Design review of the part built by this model. Coordinates are the model's own, in mm. A direction names the side the tool comes from. Give positions to 0.01 mm unless a question says otherwise; leave off trailing zeros. Order: outer loops, then holes, each group sorted by start corner. A loop starts at its lowest first (then second) coordinate and runs counter-clockwise, first axis right, second up.
```python
from build123d import *

# Parameters (mm, degrees)
SKETCH_1_W          = 38
SKETCH_1_H          = 70
SKETCH_1_R          = 1.5
SKETCH_1_W_2        = 30
SKETCH_1_H_2        = 54
SKETCH_1_H_3        = 5
EXTRUDE_1_DEPTH     = 3
EXTRUDE_2_DEPTH     = 3
FILLET_1_R          = 2
SKETCH_4_R          = 1.5
CUT_EXTRUDE_1_DEPTH = 10
FILLET_2_R          = 5


with BuildPart() as part:
    # 草图1 → 凸台-拉伸1 (new body)
    # profile 1 of 2: a face of its own
    with BuildSketch(Plane(origin=(0, 0, 0), x_dir=(1, 0, 0), z_dir=(0, 1, 0))):
        Rectangle(SKETCH_1_W, SKETCH_1_H)
        with Locations(Location((13, 31, 0), (0, 0, 270))):
            Circle(SKETCH_1_R, mode=Mode.SUBTRACT)
        with Locations(Location((-13, 31, 0), (0, 0, 270))):
            Circle(SKETCH_1_R, mode=Mode.SUBTRACT)
        with Locations(Location((9, -31, 0), (0, 0, 270))):
            Circle(SKETCH_1_R, mode=Mode.SUBTRACT)
        with Locations(Location((-9, -31, 0), (0, 0, 270))):
            Circle(SKETCH_1_R, mode=Mode.SUBTRACT)
        Rectangle(SKETCH_1_W_2, SKETCH_1_H_2, mode=Mode.SUBTRACT)
    # profile 2 of 2: a face of its own
    with BuildSketch(Plane(origin=(0, 0, 0), x_dir=(1, 0, 0), z_dir=(0, 1, 0))):
        with Locations((0, 37.5)):
            Rectangle(SKETCH_1_W, SKETCH_1_H_3)
    extrude(amount=EXTRUDE_1_DEPTH)

    # 草图2 → 凸台-拉伸2 (add)
    with BuildSketch(Plane(origin=(0, 3, 0), x_dir=(1, 0, 0), z_dir=(0, 1, 0))):
        Polygon((15, 27), (12.5, 27), (0, 4.272727273), (-12.5, 27), (-15, 27), (-15, 23), (-2.35, 0), (-15, -23), (-15, -27), (-12.5, -27), (0, -4.272727273), (12.5, -27), (15, -27), (15, -23), (2.35, 0), (15, 23), align=None)
    extrude(amount=-EXTRUDE_2_DEPTH)

    # 圆角1
    fillet_1_edges = [part.edges().sort_by_distance(p)[0] for p in [
        (-2.35, 1.5, 0),
        (-15, 1.5, -23),
        (-12.5, 1.5, -27),
        (0, 1.5, -4.272727273),
        (12.5, 1.5, -27),
        (15, 1.5, -23),
        (2.35, 1.5, 0),
        (15, 1.5, 23),
        (12.5, 1.5, 27),
        (0, 1.5, 4.272727273),
        (-12.5, 1.5, 27),
        (-15, 1.5, 23),
    ]]
    fillet(fillet_1_edges, radius=FILLET_1_R)

    # 草图4 → 切除-拉伸1 (cut)
    with BuildSketch(Plane(origin=(0, 3, 0), x_dir=(1, 0, 0), z_dir=(0, 1, 0))):
        with Locations(Location((-5, 36, 0), (0, 0, 270))):
            Circle(SKETCH_4_R)
        with Locations(Location((5, 36, 0), (0, 0, 270))):
            Circle(SKETCH_4_R)
    extrude(amount=-CUT_EXTRUDE_1_DEPTH, mode=Mode.SUBTRACT)

    # 圆角2
    fillet_2_edges = [part.edges().sort_by_distance(p)[0] for p in [
        (-19, 1.5, 35),
        (-19, 1.5, -40),
        (19, 1.5, -40),
        (19, 1.5, 35),
    ]]
    fillet(fillet_2_edges, radius=FILLET_2_R)


solid = part.part
```
1. For line 1 along X through (y, z) = (2.3, -31); line 2 along Z through (x, y) = (-9.5, 2.1); line 3 along Z through (x, y) = (12, 0.25), list the stretches that pass through material, from the lowest coordinate up.
Recorded:
line 1: x = -19 to -14.5, -11.5 to 11.5, 14.5 to 19
line 2: z = -40 to -26.96, -21.55 to -13, 13 to 21.55, 26.96 to 29.59, 32.41 to 35
line 3: z = -40 to -32.12, -29.88 to -16.95, 16.95 to 35
2. Draft analysis for pull direction Z (two halves, no side actions). For faces 3 (the face through (-18, 2, 33)), 4 (the face through (0.03, 1.479, -6.423)), 5 (the face through (-18, 2, -38)), state which applies: pulls with the +Z half, pulls with the -Z half, needs draft (parallel to the pull), parting line crosses it, or undercut.
Recorded:
face 3: pulls with the +Z half
face 4: undercut
face 5: pulls with the -Z half
3. Take a section at D-D (y = 2.55). State how many separate pieces and enclosed holes the cut face has, then the cut area to 3 significant figures.
Recorded:
separate pieces: 1
enclosed holes: 10
area: 1,690 mm2
4. For pin 1 (1.5 mm diameter, centred on x = 12.5, z = -9, fed in from -Y), flat-tipped, find the tip position at first contact; note if it passes through.
Recorded:
pin 1: passes through
5. Take a section at B-B (z = 19). State the section outline as (x, y) points, then the cut area to 3 significant figures.
Recorded:
outline: (-19, 0) - (-8.1, 0) - (-8.1, 3) - (-19, 3) - close; (8.1, 0) - (19, 0) - (19, 3) - (8.1, 3) - close
area: 65.4 mm2
6. Machinability: for faces 1 (the face through (-0.03, 1.479, 6.423)), 2 (the face through (17, 2, -39)), which of the approach directions +Z, -Z, +X, -X, +Y, -Y give a long, thin tool a straight path to every point of the face, cutting with its end or side? Answer none if there is none.
Recorded:
face 1: +Y, -Y
face 2: -Z, +X, +Y, -Y
7. Take a section at C-C (x = 13). State the section outline as (y, z) points, then the cut area to 3 significant figures.
Recorded:
outline: (0, -40) - (3, -40) - (3, -32.5) - (0, -32.5) - close; (0, -29.5) - (3, -29.5) - (3, -17.21) - (0, -17.21) - close; (0, 17.21) - (3, 17.21) - (3, 35) - (0, 35) - close
area: 113 mm2
8. Take a section at A-A (z = -31). State the section outline as (x, y) points.
Recorded:
outline: (-19, 0) - (-14.5, 0) - (-14.5, 3) - (-19, 3) - close; (-11.5, 0) - (11.5, 0) - (11.5, 3) - (-11.5, 3) - close; (14.5, 0) - (19, 0) - (19, 3) - (14.5, 3) - close
